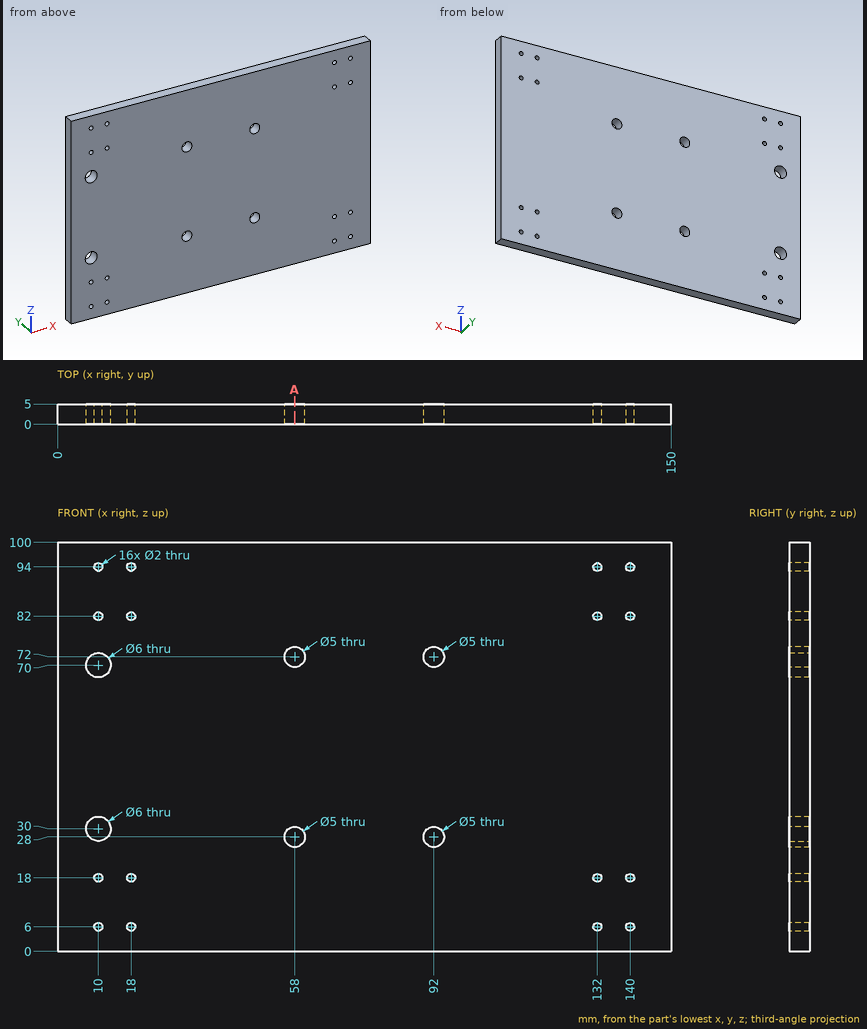
Input: dimensioned drawing with shaded views. Units: mm. Origin: part minimum x, y, z. Give positions to 0.01 mm unless a question says otherwise; leave off trailing zeros. Write each loop counter-clockwise with the first axis right and the second up, starting at its lowest first coordinate (ties: lowest second). Pieces come first, ordered by that corner, then holes.
1. Section query A-A (x = 58). Return the cut outline in (y, z).
2. Material intervals for line 1 along Z through (x, y) = (140, 3.7); line 2 along X through (y, z) = (1.45, 18); line 3 along X through (y, z) = (2.9, 30), sorted ascending.
3. First-contact query: pin 1 (1.8 mm diameter, centred on x = 10, z = 82, fed in from +Y). Flat tip, straight axial feed; report the tip coordinate or a pass-through.
Output values:
1. outline: (0, 0) - (5, 0) - (5, 25.5) - (0, 25.5) - close; (0, 30.5) - (5, 30.5) - (5, 69.5) - (0, 69.5) - close; (0, 74.5) - (5, 74.5) - (5, 100) - (0, 100) - close
2. line 1: z = 0 to 5, 7 to 17, 19 to 81, 83 to 93, 95 to 100
2. line 2: x = 0 to 9, 11 to 17, 19 to 131, 133 to 139, 141 to 150
2. line 3: x = 0 to 7, 13 to 56.5, 59.5 to 90.5, 93.5 to 150
3. pin 1: passes through
